Here's how the part is built. I have some questions about the finished solid (model axes, mm). Face numbers are marked on the shaded views. A direction names the side the tool comes from. Round coordinates to 2 decimals unless told otherwise and drop trailing zeros. Order: outer loops, then holes, each group sorted by start corner. A loop starts at its lowest first (then second) coordinate and runs counter-clockwise, first axis right, second up. Notation, with made-up numbers: (-40, 68.5) -> (-14, 68.5) arc R24 cw to (-14, 83.5) -> close; hole circle Ø11 at (87, 17). An arc over 180 degrees is marked (long way). Use a Markdown table: item, result. Add a question column.
(1) On a 3-axis mill with a long thin cutter (end or side, diameter ignored), from which of +Z, -Z, +X, -X, +Y, -Y can I reach the whole of each face in a straight line? I mean the marked faces 1, 2 and 3. Say none if no direction works.
(2) Thinking about a two-plate mould opening in X: for the marked faces 4, 5, 6 and 7, which applies, pulls with the +X half, pulls with the -X half, needs draft (parallel to the pull), parting line crosses it, or undercut?
(3) I want a section at C-C, the plane y = 4. Please give me the cut outline in (x, z), then the cut area to 3 significant figures.
(4) I want a section at A-A, the plane z = 10.75. Please give me the cut outline in (x, y), then the cut area to 3 significant figures.
(5) I'm going to push flat-ended pins straight in: P1, Ø3.5, axis at x = 8.86, y = 8.05, coming from the -Z side; P2, Ø1, axis at x = 21.5, z = 6.5, coming from the -Y side; P3, Ø4, axis at y = -5.5, z = 6.5, coming from the +X side; P4, Ø4, axis at x = 6.5, z = 8, coming from the -Y side. Where does each tip first touch, or does it pass through?
(6) If I drill on probe 1 along X at (y, z) = (-4.5, 3); probe 2 along X at (y, z) = (-1.25, 6); probe 3 along X at (y, z) = (9, 1.5), over which ranges is the centre line in solid material (lowest first)?
(7) I want a section at B-B, the plane y = 10.5. Please give me the cut outline in (x, z).
(8) I want a section at D-D, the plane x = 11.5. Please give me the cut outline in (y, z).
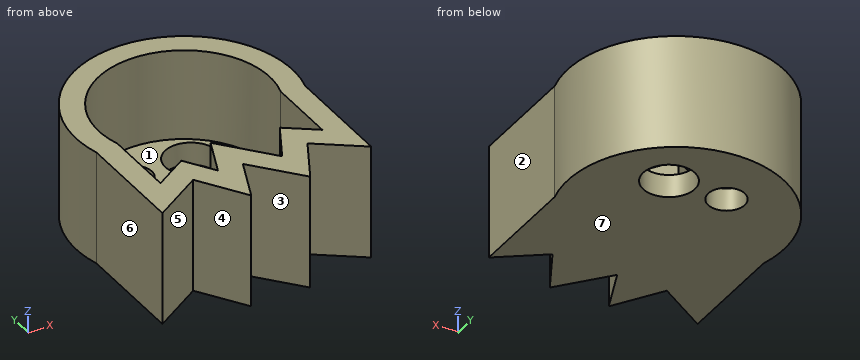
from build123d import *

# Parameters (mm, degrees)
F0_R     = 2.7361365436
F0_R_2   = 5.9630121177
F1_DEPTH = 12.7
F3_T     = -2.54
F2_R     = 2.8890765553
F2_R_2   = 2.0489311255
F4_DEPTH = 61.976


with BuildPart() as f1:
    # F0 (on Top) → F1 (new body)
    with BuildSketch(Plane.XY):
        with BuildLine():
            Line((23.336250335, -12.5060621649), (23.336250335, 0))
            ThreePointArc((23.336250335, 0), (11.6681251675, 15.2751887217), (0, 0))
            Line((0, 0), (0, -12.5060621649))
            Line((0, -12.5060621649), (5.556251388, -8.8944993913))
            Line((5.556251388, -8.8944993913), (8.9647026685, -14.1382715047))
            Line((8.9647026685, -14.1382715047), (11.1124990508, -8.8944993913))
            Line((11.1124990508, -8.8944993913), (15.5575014651, -14.1382715047))
            Line((15.5575014651, -14.1382715047), (18.3356255293, -8.8944993913))
            Line((18.3356255293, -8.8944993913), (23.336250335, -12.5060621649))
        make_face()
        with Locations((4.4449996203, 4.1626878083)):
            Circle(F0_R, mode=Mode.SUBTRACT)
        with Locations((15.5575014651, 4.7183129936)):
            Circle(F0_R_2, mode=Mode.SUBTRACT)
        with Locations((15.5575014651, 4.7183129936)):
            Circle(F0_R_2)
        with Locations((4.4449996203, 4.1626878083)):
            Circle(F0_R)
    extrude(amount=F1_DEPTH)

    # F3
    f3_openings = [f1.faces().sort_by_distance(p)[0] for p in [
        (11.684831, 0.988921, 12.7),
    ]]
    offset(amount=F3_T, openings=f3_openings, kind=Kind.INTERSECTION)

    # F2 (on Top) → F4 (cut)
    with BuildSketch(Plane.XY):
        with Locations((15.2920437977, 8.0478740856)):
            Circle(F2_R)
        with Locations((8.8641922921, 8.0478740856)):
            Circle(F2_R_2)
    extrude(amount=F4_DEPTH, mode=Mode.SUBTRACT)


solid = f1.part
Taken from the geometry:
| question | item | result |
|---|---|---|
| 1 | face 1 | +Z |
| 1 | face 2 | +Z, -Z, +X, -Y |
| 1 | face 3 | +Z, -Z, -Y |
| 2 | face 4 | undercut |
| 2 | face 5 | undercut |
| 2 | face 6 | pulls with the -X half |
| 2 | face 7 | needs draft |
| 3 | outline | (-0.4, 0) -> (23.73, 0) -> (23.73, 12.7) -> (21.19, 12.7) -> (21.19, 2.54) -> (2.15, 2.54) -> (2.15, 12.7) -> (-0.4, 12.7) -> close |
| 3 | area | 113 mm2 |
| 4 | outline | (0, -12.51) -> (5.56, -8.89) -> (8.96, -14.14) -> (11.11, -8.89) -> (15.56, -14.14) -> (18.34, -8.89) -> (23.34, -12.51) -> (23.34, 0) arc R12.09 ccw (long way) to (0, 0) -> close; hole (2.54, -7.83) -> (6.3, -5.38) -> (8.45, -8.69) -> (10.35, -4.06) -> (15.07, -9.63) -> (17.46, -5.13) -> (20.8, -7.54) -> (20.8, 0.36) arc R9.55 ccw (long way) to (2.54, 0.36) -> close |
| 4 | area | 240 mm2 |
| 5 | P1 | passes through |
| 5 | P2 | stops at y = -11.54 |
| 5 | P3 | stops at x = 23.34 |
| 5 | P4 | stops at y = -13.42 |
| 6 | probe 1 | x = 0 to 2.54, 10.17 to 10.72, 20.8 to 23.34 |
| 6 | probe 2 | x = 0 to 2.54, 20.8 to 23.34 |
| 6 | probe 3 | x = 1.07 to 7.05, 10.68 to 12.56, 18.02 to 22.27 |
| 7 | outline | (2.04, 0) -> (13.76, 0) -> (13.76, 2.54) -> (5.53, 2.54) -> (5.53, 12.7) -> (2.04, 12.7) -> close; (16.82, 0) -> (21.3, 0) -> (21.3, 12.7) -> (17.81, 12.7) -> (17.81, 2.54) -> (16.82, 2.54) -> close |
| 8 | outline | (-9.35, 0) -> (15.27, 0) -> (15.27, 12.7) -> (12.73, 12.7) -> (12.73, 2.54) -> (-5.42, 2.54) -> (-5.42, 12.7) -> (-9.35, 12.7) -> close |
